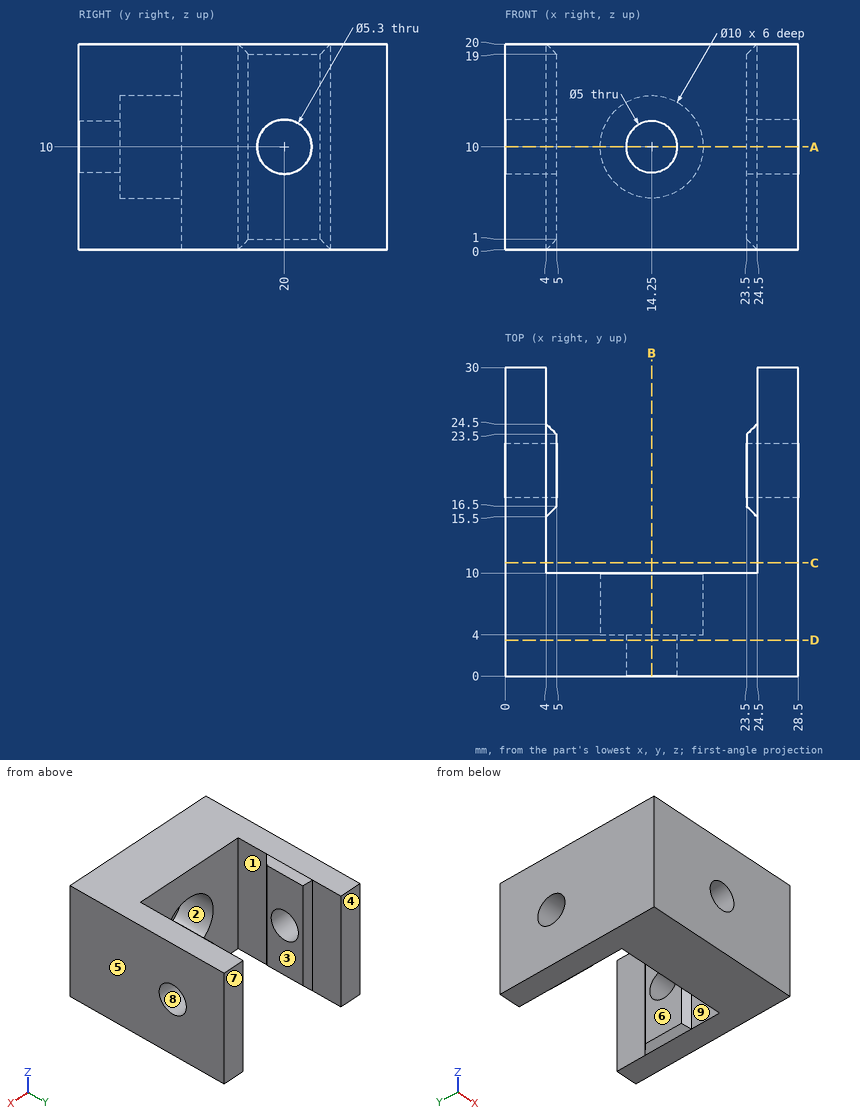
Could you check a few things on this drawing? It's one solid part, dimensions in mm from its lowest x, y, z. A direction names the side the tool comes from. Coordinates: 2 decimals unless noted, no trailing zeros. Order: outer loops, then holes, each group sorted by start corner. A loop starts at its lowest first (then second) coordinate and runs counter-clockwise, first axis right, second up. Notation, with made-up numbers: M -13,-8.5 L 5,-8.5 A20 cw 5,24.5 Z; hole C -9,-11.5 d1. An arc over 180 degrees is marked long. Use one line per item in the form item = value. Start each with the question number.
1. Suppose I cut it at A-A on z = 10. Count the separate pieces of the cut face and the enclosed holes in it, then the cut area to 3 significant figures.
2. Suppose I cut it at C-C on y = 11. Write out the boundary of the cut face in (x, z).
3. Please list where these lines run through material, in increasing order: line 1 (X direction, y = 28, z = 4); line 2 (Z direction, x = 26.8, y = 20); line 3 (Z direction, x = 14.25, y = 0.8).
4. Suppose I cut it at D-D on y = 3.5. Write out the boundary of the cut face in (x, z).
5. For pin 1 (5 mm diameter, centred on y = 21.5, z = 16.5, fed in from -X); pin 2 (6 mm diameter, centred on x = 9.5, z = 7.5, fed in from +Y); pin 3 (8 mm diameter, centred on x = 14.25, z = 10, fed in from +Y), each with a flat end and sliding along its axis, tell me the tip position at first contact or that it passes through.
6. On a 3-axis mill with a long thin cutter (end or side, diameter ignored), from which of +Z, -Z, +X, -X, +Y, -Y can I reach the whole of each face in a straight line? I mean the marked faces 1, 2, 3, 4 and 5. Say none if no direction works.
7. We'd pull the mould along Y, two halves only. Please class the marked faces 6, 7, 8 and 9: +Y half, -Y half, draft (parallel to the pull), parting line (faces both ways), or undercut.
8. Suppose I cut it at B-B on x = 14.25. Write out the boundary of the cut face in (y, z), then the cut area to 3 significant figures.
Geometry says:
q1.separate_pieces = 4
q1.enclosed_holes = 0
q1.area = 328 mm^2
q2.outline = M 0,0 L 4,0 L 4,20 L 0,20 Z; M 24.5,0 L 28.5,0 L 28.5,20 L 24.5,20 Z
q3.line_1 = 0 to 4, 24.5 to 28.5
q3.line_2 = 0 to 7.35, 12.65 to 20
q3.line_3 = 0 to 7.5, 12.5 to 20
q4.outline = M 0,0 L 28.5,0 L 28.5,20 L 0,20 Z; hole C 14.25,10 d5
q5.pin_1 = 0
q5.pin_2 = 10
q5.pin_3 = 4
q6.face_1 = +Z, -Z
q6.face_2 = +Y
q6.face_3 = +Z, -Z, +Y
q6.face_4 = +Z, -Z, +X, -X, +Y
q6.face_5 = +Z, -Z, +X, +Y, -Y
q7.face_6 = draft
q7.face_7 = +Y half
q7.face_8 = undercut
q7.face_9 = undercut
q8.outline = M 0,0 L 10,0 L 10,5 L 4,5 L 4,7.5 L 0,7.5 Z; M 0,12.5 L 4,12.5 L 4,15 L 10,15 L 10,20 L 0,20 Z
q8.area = 120 mm^2
